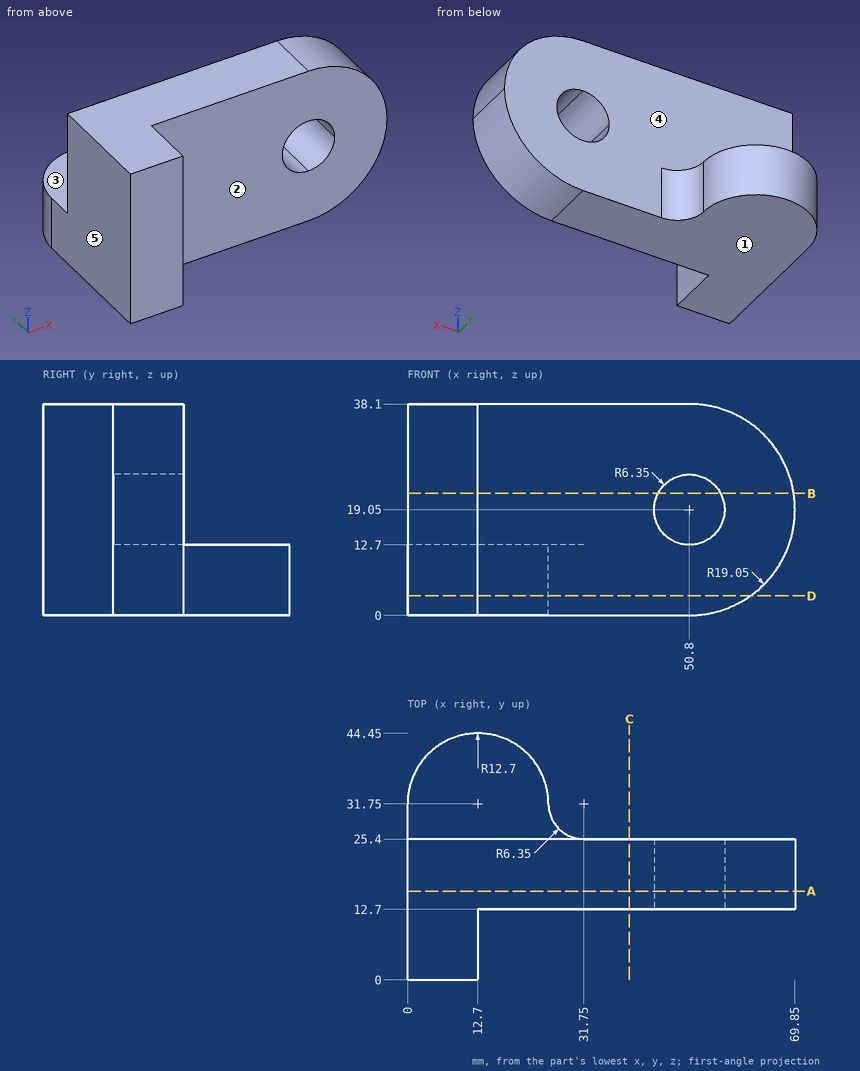
Print and shaded views of the part. All mm, measured from the part's lowest x, y and z. A direction names the side the tool comes from. Round coordinates to 2 decimals unless told otherwise and drop trailing zeros. Write each loop counter-clockwise with the first axis right and the second up, starting at its lowest first coordinate (ties: lowest second). Pieces come first, ordered by that corner, then holes. Notation, with made-up numbers: (22.5, -39.5) -> (65.5, -39.5) arc R23 ccw to (65.5, -25.5) -> close; hole circle Ø1 at (39, -16.5). An arc over 180 degrees is marked (long way). Return JSON: item names as keys, results as strings. Group by question number.
Q1. Saw through at A-A on y = 16. Write the cut outline in (x, z), plus the area to 3 significant figures.
Q2. Pin check, flat tips, straight feed: pin 1 (2 mm diameter, centred on y = 36, z = 5, fed in from -X); pin 2 (11.5 mm diameter, centred on x = 31.5, z = 14.5, fed in from -Y); pin 3 (12 mm diameter, centred on x = 41.5, y = 6, fed in from -Z); pin 4 (10 mm diameter, centred on y = 8.5, z = 13.5, fed in from +X). Stop position of each tip, or through.
Q3. Saw through at C-C on x = 40. Write the cut outline in (y, z), plus the area to 3 significant figures.
Q4. Saw through at B-B on z = 22. Write the cut outline in (x, y), plus the area to 3 significant figures.
Q5. Which spindle directions (+Z, -Z, +X, -X, +Y, -Y) get a long thin tool onto all of the face, cutting with end or side? Do the marked faces 1, 2, 3, 4 and 5. Say none if no direction does.
Q6. Probe L1, parallel to Y at x = 49, z = 34; L2, parallel to Z at x = 12, y = 31; L3, parallel to X at y = 13, z = 23.5. List the from-to ranges inside material, lowest first. Write a range as [from, to].
Q7. Saw through at D-D on z = 3.5. Write the cut outline in (x, y), plus the area to 3 significant figures.
Answer:
{
 "1": {"outline": "(0, 0) -> (50.8, 0) arc R19.05 ccw to (50.8, 38.1) -> (0, 38.1) -> close; hole circle Ø12.7 at (50.8, 19.05)", "area": "2,380 mm2"},
 "2": {"pin 1": "x = 0.42", "pin 2": "y = 12.7", "pin 3": "through", "pin 4": "x = 69.64"},
 "3": {"outline": "(12.7, 0) -> (25.4, 0) -> (25.4, 38.1) -> (12.7, 38.1) -> close", "area": "484 mm2"},
 "4": {"outline": "(0, 0) -> (12.7, 0) -> (12.7, 12.7) -> (45.18, 12.7) -> (45.18, 25.4) -> (0, 25.4) -> close; (56.42, 12.7) -> (69.62, 12.7) -> (69.62, 25.4) -> (56.42, 25.4) -> close", "area": "903 mm2"},
 "5": {"face 1": "-Z, +X, -X, +Y, -Y", "face 2": "+Z, -Z, +X, -Y", "face 3": "+Z, +X, -X, +Y", "face 4": "+Z, +X, +Y", "face 5": "+Z, -Z, -X, +Y, -Y"},
 "6": {"L1": "[12.7, 25.4]", "L2": "[0, 12.7]", "L3": "[0, 46.27], [55.33, 69.32]"},
 "7": {"outline": "(0, 0) -> (12.7, 0) -> (12.7, 12.7) -> (61.8, 12.7) -> (61.8, 25.4) -> (31.75, 25.4) arc R6.35 cw to (25.4, 31.75) arc R12.7 ccw to (0, 31.75) -> close", "area": "1,370 mm2"}
}
